Input: part model. Units: mm. Frame: model coordinates. Face numbers are marked on the shaded views. Round coordinates to 2 decimals unless told otherwise and drop trailing zeros. Loops run counter-clockwise (first coordinate to the right, second up) from the corner with the lowest first, then second, coordinate; pieces in that order, holes last.
1) Section B-B, the plane x = 0. Return loops of the section in (y, z), and give its area (3 significant figures).
2) First-contact query: pin 1 (5 mm diameter, centred on x = -2, z = 52.5, fed in from -Y); pin 2 (12 mm diameter, centred on x = 1, y = -61, fed in from +Z); pin 3 (8 mm diameter, centred on x = 26, z = 7, fed in from +Y); pin 4 (3 mm diameter, centred on y = -33, z = -11, fed in from +X). Flat tips, straight axial feed; report the tip coordinate or a pass-through.
3) Section C-C, the plane y = -8.5. Return loops of the section in (x, z).
4) Section A-A, the plane z = 0. Return loops of the section in (x, y), and give its area (3 significant figures).
5) Draft query along Z for the marked faces 1, 2, 3 and 4. Return one class per face: pulls with the +Z half, pulls with the -Z half, needs draft (parallel to the pull), parting line crosses it, or undercut.
6) Ray query, line 1 along Z through (x, y) = (0, -63); line 2 along X through (y, z) = (-0.55, 0). Return the intervals inside material, ascending.
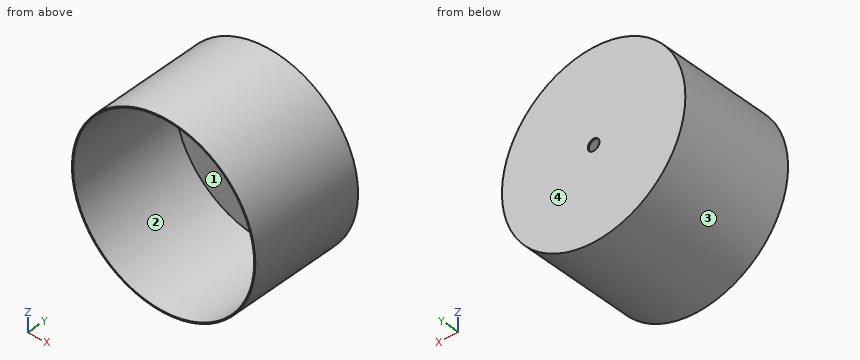
from build123d import *

# Parameters (mm, degrees)
SKETCH1_R           = 77.5
BOSS_EXTRUDE1_DEPTH = 1
SKETCH1_2_R         = 78.5
SKETCH1_2_R_2       = 77.5
EXTRUDE_THIN1_DEPTH = 100
SKETCH2_R           = 5
CUT_EXTRUDE1_DEPTH  = 101


with BuildPart() as part:
    # Sketch1 → Boss-Extrude1 (new body)
    with BuildSketch(Plane(origin=(0, 0, 0), x_dir=(1, 0, 0), z_dir=(0, 1, 0))):
        Circle(SKETCH1_R)
    extrude(amount=-BOSS_EXTRUDE1_DEPTH)

    # Sketch1<2> → Extrude-Thin1 (add)
    with BuildSketch(Plane(origin=(0, 0, 0), x_dir=(1, 0, 0), z_dir=(0, 1, 0))):
        Circle(SKETCH1_2_R)
        Circle(SKETCH1_2_R_2, mode=Mode.SUBTRACT)
    extrude(amount=-EXTRUDE_THIN1_DEPTH)

    # Sketch2 → Cut-Extrude1 (cut, through all)
    with BuildSketch(Plane(origin=(0, 0, 0), x_dir=(1, 0, 0), z_dir=(0, 1, 0))):
        Circle(SKETCH2_R)
    extrude(amount=-CUT_EXTRUDE1_DEPTH, mode=Mode.SUBTRACT)


solid = part.part
Final values:
1. outline: (-100, -78.5) - (0, -78.5) - (0, -5) - (-1, -5) - (-1, -77.5) - (-100, -77.5) - close; (-100, 77.5) - (-1, 77.5) - (-1, 5) - (0, 5) - (0, 78.5) - (-100, 78.5) - close
1. area: 345 mm2
2. pin 1: stops at y = -1
2. pin 2: stops at z = 78.5
2. pin 3: stops at y = 0
2. pin 4: stops at x = 77.92
3. outline: circle Ø157 at (0, 0); hole circle Ø155 at (0, 0)
4. outline: (-78.5, -100) - (-77.5, -100) - (-77.5, -1) - (-5, -1) - (-5, 0) - (-78.5, 0) - close; (5, -1) - (77.5, -1) - (77.5, -100) - (78.5, -100) - (78.5, 0) - (5, 0) - close
4. area: 345 mm2
5. face 1: undercut
5. face 2: undercut
5. face 3: parting line crosses it
5. face 4: needs draft
6. line 1: z = -78.5 to -77.5, 77.5 to 78.5
6. line 2: x = -78.5 to -5, 5 to 78.5
